CAD build for the part. Positions are in the model's coordinates, mm. A direction names the side the tool comes from. Give positions to 0.01 mm unless a question says otherwise; leave off trailing zeros. Order: outer loops, then holes, each group sorted by start corner. A loop starts at its lowest first (then second) coordinate and runs counter-clockwise, first axis right, second up. Notation, with made-up numbers: (-31, -4) -> (-9, -4) arc R17 cw to (-9, 28) -> close; hole circle Ø3 at (86, 50.25). An arc over 180 degrees is marked (long way). Answer as CSV lines item,"result".
```python
from build123d import *

# Parameters (mm, degrees)
SKETCH1_W            = 150
SKETCH1_H            = 1.5
BOSS_EXTRUDE1_DEPTH  = 190
BOSS_EXTRUDE2_DEPTH  = 10
BOSS_EXTRUDE3_START  = 3
SKETCH3_R            = 1.4
BOSS_EXTRUDE3_DEPTH  = 3
FILLET1_R            = 1
FILLET2_R            = 10
FILLET1_OF_MIRROR2_R = 1
FILLET2_OF_MIRROR2_R = 10
LPATTERN1_START      = 175.9999999
LPATTERN1_OUTLINE_R  = 1.4
LPATTERN1_DEPTH      = 12.0000001
LPATTERN1_START_2    = 178
LPATTERN1_2_DEPTH    = 10


with BuildPart() as part:
    # Sketch1 → Boss-Extrude1 (new body)
    with BuildSketch(Plane(origin=(0, 0, 0), x_dir=(1, 0, 0), z_dir=(0, 1, 0))):
        Rectangle(SKETCH1_W, SKETCH1_H)
    extrude(amount=BOSS_EXTRUDE1_DEPTH)

    # Sketch2 → Boss-Extrude2 (add)
    with BuildSketch(Plane(origin=(0, 8, 0), x_dir=(1, 0, 0), z_dir=(0, 1, 0))):
        with BuildLine():
            Line((-75, 0.75), (-77.993576193, 2.550233244))
            ThreePointArc((-77.993576193, 2.550233244), (-78.48384028, 4.451164765), (-76.591446047, 4.973413351))
            Line((-76.591446047, 4.973413351), (-69, 0.75))
            Line((-69, 0.75), (-75, 0.75))
        make_face()
    boss_extrude2 = extrude(amount=BOSS_EXTRUDE2_DEPTH)

    # Sketch3 → Boss-Extrude3 (add)
    with BuildSketch(Plane(origin=(0, 8, 0), x_dir=(-1, 0, 0), z_dir=(0, -1, 0)).offset(BOSS_EXTRUDE3_START)):
        with Locations(Location((77.272077939, 3.75, 0), (0, 0, 180))):
            Circle(SKETCH3_R)
    boss_extrude3 = extrude(amount=-BOSS_EXTRUDE3_DEPTH)

    # Fillet1
    fillet1_edges = [part.edges().sort_by_distance(p)[0] for p in [
        (-78.672077939, 5, -3.75),
    ]]
    fillet(fillet1_edges, radius=FILLET1_R)

    # Fillet2
    fillet2_edges = [part.edges().sort_by_distance(p)[0] for p in [
        (-69, 13, -0.75),
    ]]
    fillet(fillet2_edges, radius=FILLET2_R)

    # Mirror2: Boss-Extrude2, Boss-Extrude3 across plane
    add(boss_extrude2.mirror(Plane(origin=(0, 0, 0), x_dir=(0, 0, 1), z_dir=(1, 0, 0))))
    add(boss_extrude3.mirror(Plane(origin=(0, 0, 0), x_dir=(0, 0, 1), z_dir=(1, 0, 0))))

    # Fillet1 of Mirror2
    fillet1_of_mirror2_edges = [part.edges().sort_by_distance(p)[0] for p in [
        (78.672077939, 5, -3.75),
    ]]
    fillet(fillet1_of_mirror2_edges, radius=FILLET1_OF_MIRROR2_R)

    # Fillet2 of Mirror2
    fillet2_of_mirror2_edges = [part.edges().sort_by_distance(p)[0] for p in [
        (69, 13, -0.75),
    ]]
    fillet(fillet2_of_mirror2_edges, radius=FILLET2_OF_MIRROR2_R)



with BuildPart() as body_2:
    # LPattern1: read off the stored shape, not the designer's step
    # LPattern1 outline → LPattern1 (new body)
    with BuildSketch(Plane(origin=(0, 0, 0), x_dir=(1, 0, 0), z_dir=(0, 1, 0)).offset(LPATTERN1_START)):
        with Locations((-77.272077939, 3.75)):
            Circle(LPATTERN1_OUTLINE_R)
        with Locations((77.272077939, 3.75)):
            Circle(LPATTERN1_OUTLINE_R)
    extrude(amount=LPATTERN1_DEPTH)


with BuildPart() as part_1:
    add(part.part)

    add(body_2.part)  # LPattern1 2 merges body 2
    # LPattern1 2 outline → LPattern1 2 (add)
    with BuildSketch(Plane(origin=(0, 0, 0), x_dir=(1, 0, 0), z_dir=(0, 1, 0)).offset(LPATTERN1_START_2)):
        with BuildLine():
            ThreePointArc((71.267204788, 2.011333205), (68.916856052, 1.070468298), (66.40554842, 0.75))
            Line((66.40554842, 0.75), (75, 0.75))
            Line((75, 0.75), (77.993576193, 2.550233244))
            ThreePointArc((77.993576193, 2.550233244), (76.060315597, 3.048835235), (76.591446047, 4.973413351))
            Line((76.591446047, 4.973413351), (71.267204788, 2.011333205))
        make_face()
        with BuildLine():
            Line((-71.267204788, 2.011333205), (-76.591446047, 4.973413351))
            ThreePointArc((-76.591446047, 4.973413351), (-76.060315597, 3.048835235), (-77.993576193, 2.550233244))
            Line((-77.993576193, 2.550233244), (-75, 0.75))
            Line((-75, 0.75), (-66.40554842, 0.75))
            ThreePointArc((-66.40554842, 0.75), (-68.916856052, 1.070468298), (-71.267204788, 2.011333205))
        make_face()
    extrude(amount=LPATTERN1_2_DEPTH)

    # LPattern1 3 outline → LPattern1 3 (revolve)
    with BuildSketch(Plane(origin=(77.272077939, 0, -3.75), x_dir=(1, 0, 0), z_dir=(0, 0, 1))):
        with BuildLine():
            Line((0, 175.9999999), (0, 175))
            Line((0, 175), (0.4, 175))
            ThreePointArc((0.4, 175), (1.107106781, 175.292893219), (1.4, 176))
            Line((1.4, 176), (0, 175.9999999))
        make_face()
    revolve(axis=Axis((77.272077939, 0, -3.75), (0, 1, 0)))

    # LPattern1 4 outline → LPattern1 4 (revolve)
    with BuildSketch(Plane(origin=(-77.272077939, 0, -3.75), x_dir=(1, 0, 0), z_dir=(0, 0, 1))):
        with BuildLine():
            Line((0, 175.9999999), (0, 175))
            Line((0, 175), (0.4, 175))
            ThreePointArc((0.4, 175), (1.107106781, 175.292893219), (1.4, 176))
            Line((1.4, 176), (0, 175.9999999))
        make_face()
    revolve(axis=Axis((-77.272077939, 0, -3.75), (0, 1, 0)))


solid = part_1.part
```
1) Pin check, flat tips, straight feed: P1, Ø3.5, axis at x = 73.5, z = -3, coming from the +Y side; P2, Ø10, axis at x = 34, y = 105, coming from the -Z side; P3, Ø3, axis at x = -43, z = -1, coming from the -Y side; P4, Ø2, axis at x = -73.5, z = -3.5, coming from the -Y side. Stop position of each tip, or through.
Data:
P1,"stops at y = 188"
P2,"stops at z = -0.75"
P3,"stops at y = 0"
P4,"stops at y = 8"
2) Band-saw the part on A-A, the plane y = 14. Write the cut outline in (x, z), then the cut area to 3 significant figures.
Data:
outline,"(-77.99, -2.55) arc R1.4 ccw to (-76.59, -4.97) -> (-71.27, -2.01) arc R10 cw to (-66.41, -0.75) -> (66.41, -0.75) arc R10 cw to (71.27, -2.01) -> (76.59, -4.97) arc R1.4 ccw to (77.99, -2.55) -> (75, -0.75) -> (75, 0.75) -> (-75, 0.75) -> (-75, -0.75) -> close"
area,"267 mm2"
3) Band-saw the part on B-B, the plane x = -38. Write the cut outline in (y, z), then the cut area to 3 significant figures.
Data:
outline,"(0, -0.75) -> (190, -0.75) -> (190, 0.75) -> (0, 0.75) -> close"
area,"285 mm2"
4) Wall check: line 1 along Z through (x, y) = (40.5, 167); line 2 along X through (y, z) = (102, -0.05); line 3 along X through (y, z) = (180, -4.15). Give the ranges that are in metal, low to high. Write a range as [from, to].
Data:
line 1,"z = [-0.75, 0.75]"
line 2,"x = [-75, 75]"
line 3,"x = [-78.61, -75.11], [75.11, 78.61]"
5) Which spindle directions (+Z, -Z, +X, -X, +Y, -Y) get a long thin tool onto all of the face, cutting with end or side? Do faces 1 (the flat face through (75, 188, -2)), 2 (the flat face through (75, 18, -2)), 3 (the flat face through (-1, 94, 0.75)), 4 (the flat face through (73.967, 12.93, -3.513)). Say none if no direction does.
Data:
face 1,"-Z, +X, -X, +Y"
face 2,"-Z, +X, -X"
face 3,"+Z, +X, -X, +Y, -Y"
face 4,"-Z, +Y, -Y"
6) Pull direction Y, two halves, no side cores. Call faces 5 (the flat face through (74, 178, -2)), 6 (the flat face through (73.967, 182.93, -3.513)), 7 (the flat face through (74, 8, -2)), 8 (the flat face through (-75, 18, -2)): pulls with the +Y half, pulls with the -Y half, needs draft (parallel to the pull), parting line crosses it, or undercut.
Data:
face 5,"undercut"
face 6,"needs draft"
face 7,"pulls with the -Y half"
face 8,"undercut"
